Part print with two shaded views. Sizes in mm from the minimum x, y, z corner. A direction names the side the tool comes from. Coordinates: 2 decimals unless noted, no trailing zeros. Write each loop counter-clockwise with the first axis right and the second up, starting at its lowest first coordinate (ties: lowest second). Pieces come first, ordered by that corner, then holes.
Q1. Band-saw the part on A-A, the plane x = 47. Write the cut outline in (y, z).
Q2. Band-saw the part on C-C, the plane z = 8. Write the cut outline in (x, y) (1 decimal).
Q3. Band-saw the part on B-B, the plane y = 10. Write the cut outline in (x, z), plus the area to 3 significant figures.
Q4. Pull direction X, two halves, no side cores. Call the marked faces 4, 5, 6 and 7: released by +X, released by -X, zero draft, split by the parting line, or undercut.
Q5. Which spindle directions (+Z, -Z, +X, -X, +Y, -Y) get a long thin tool onto all of the face, cutting with end or side? Do the marked faces 1, 2 and 3. Say none if no direction does.
Q6. Drill centre lines: probe 1 along Y at (x, z) = (47, 7); probe 2 along X at (y, z) = (16, 12) (1 decimal); probe 3 along Z at (x, y) = (14, 26). Where is each one in solid material? Low to high.
Q7. Pin check, flat tips, straight feed: P1, Ø2, axis at x = 1, z = 6.5, coming from the +Y side; P2, Ø8, axis at y = 31, z = 5.5, coming from the -X side; P3, Ø15, axis at x = 35, y = 18, coming from the +Z side; P4, Ø14, axis at x = 13, y = 16.5, coming from the +Z side. Stop position of each tip, or through.
Q8. Band-saw the part on D-D, the plane y = 45. Write the cut outline in (x, z), plus the area to 3 significant figures.
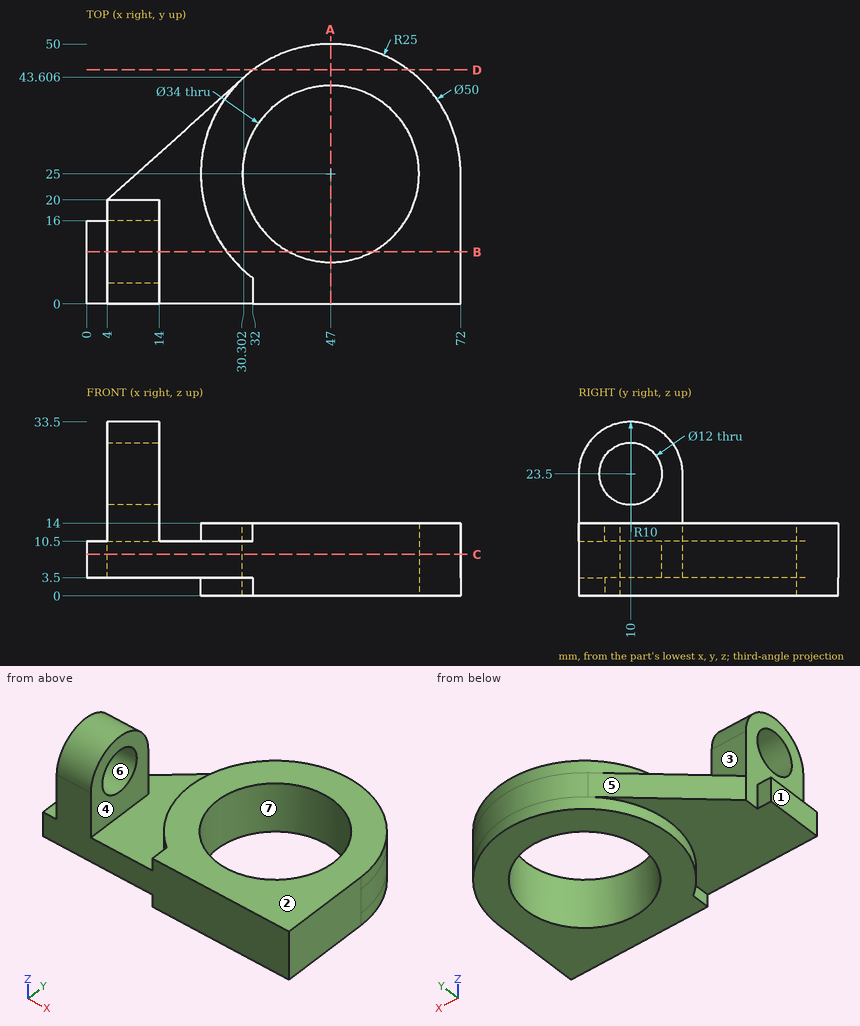
Answer sheet:
1. outline: (0, 0) - (8, 0) - (8, 14) - (0, 14) - close; (42, 0) - (50, 0) - (50, 14) - (42, 14) - close
2. outline: (0, 0) - (72, 0) - (72, 25) arc R25 ccw to (30.3, 43.6) - (4, 20) - (4, 16) - (0, 16) - close; hole circle Ø34 at (47, 25)
3. outline: (0, 3.5) - (27, 3.5) - (27, 0) - (39, 0) - (39, 14) - (27, 14) - (27, 10.5) - (14, 10.5) - (14, 17.5) - (4, 17.5) - (4, 10.5) - (0, 10.5) - close; (4, 29.5) - (14, 29.5) - (14, 33.5) - (4, 33.5) - close; (55, 0) - (72, 0) - (72, 14) - (55, 14) - close
3. area: 705 mm2
4. face 4: undercut
4. face 5: released by -X
4. face 6: zero draft
4. face 7: undercut
5. face 1: +Z, -Z, -X, +Y, -Y
5. face 2: +Z, +X, +Y, -Y
5. face 3: +Z, -X, +Y
6. probe 1: y = 0 to 8, 42 to 50
6. probe 2: x = 4 to 14, 23.7 to 32.6, 61.4 to 72
6. probe 3: z = 3.5 to 10.5
7. P1: stops at y = 16
7. P2: stops at x = 11.8
7. P3: stops at z = 14
7. P4: stops at z = 33.5
8. outline: (32, 0) - (62, 0) - (62, 14) - (32, 14) - close
8. area: 420 mm2
